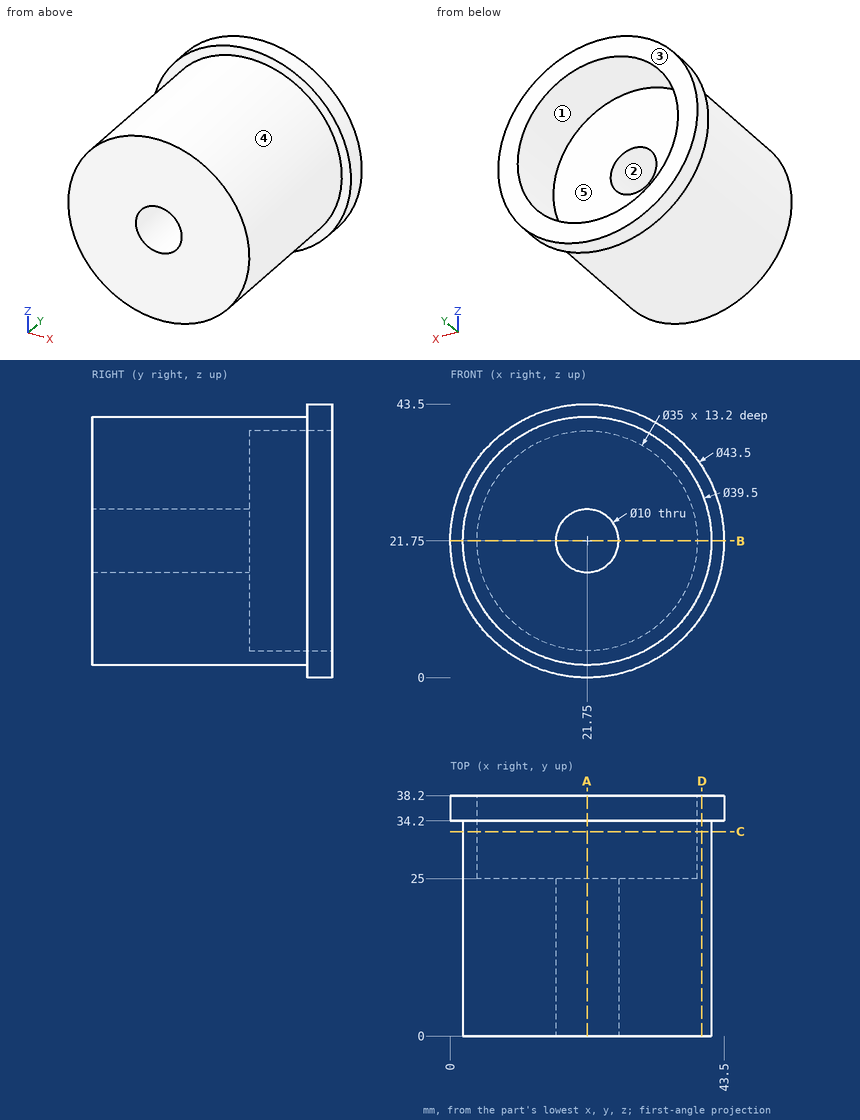
Geometry check sheet. Reference: drawing and pictorial views, mm from the part's lowest x, y, z. A direction names the side the tool comes from. Give positions to 0.01 mm unless a question says otherwise; leave off trailing zeros. Loops run counter-clockwise (first coordinate to the right, second up) from the corner with the lowest first, then second, coordinate; pieces in that order, holes last. Notation, with made-up numbers: (43.25, -25.5) - (101.25, -25.5) arc R17 ccw to (101.25, -16.5) - close; hole circle Ø9 at (85.5, -20). An arc over 180 degrees is marked (long way). Use CSV: the item, a comma, the result in double quotes. Start each with the question number.
Q1. Section check D-D, the plane x = 40. Record the cut outline in (y, z).
Q2. Section check B-B, the plane z = 21.75. Record the cut outline in (x, y).
Q3. Section check C-C, the plane y = 32.5. Record the cut outline in (x, z), and give its area (3 significant figures).
Q4. Section check A-A, the plane x = 21.75. Record the cut outline in (y, z).
Q5. Scan lines: probe 1 along X at (y, z) = (31, 21.75); probe 2 along Y at (x, z) = (31, 14); probe 3 along X at (y, z) = (3.5, 22). Record each from-to range of solid material in increasing order. Write a range as from..to.
Q6. Release check for a two-part mould opening along X. For the marked faces 3, 4 and 5 record: +X half, -X half, draft (parallel to the pull), parting line (faces both ways), or undercut.
Q7. Go/stop test with flat-tipped pins: pin 1 Ø6 at (x, y) = (33, 34) entering from -Z; pin 2 Ø1 at (x, y) = (24.5, 7) entering from +Z; pin 3 Ø5 at (y, z) = (15, 9.5) entering from +X. Record where each tip stops, or that it passes through.
Q8. Access from +Z, -Z, +X, -X, +Y, -Y to the whole of each face (thin tool, end or side, straight path). Record for the marked faces 1 and 2.
Findings below:
1,outline,"(0, 14.2) - (34.2, 14.2) - (34.2, 9.92) - (38.2, 9.92) - (38.2, 33.58) - (34.2, 33.58) - (34.2, 29.3) - (0, 29.3) - close"
2,outline,"(0, 34.2) - (2, 34.2) - (2, 0) - (16.75, 0) - (16.75, 25) - (4.25, 25) - (4.25, 38.2) - (0, 38.2) - close; (26.75, 0) - (41.5, 0) - (41.5, 34.2) - (43.5, 34.2) - (43.5, 38.2) - (39.25, 38.2) - (39.25, 25) - (26.75, 25) - close"
3,outline,"circle Ø39.5 at (21.75, 21.75); hole circle Ø35 at (21.75, 21.75)"
3,area,"263 mm^2"
4,outline,"(0, 2) - (34.2, 2) - (34.2, 0) - (38.2, 0) - (38.2, 4.25) - (25, 4.25) - (25, 16.75) - (0, 16.75) - close; (0, 26.75) - (25, 26.75) - (25, 39.25) - (38.2, 39.25) - (38.2, 43.5) - (34.2, 43.5) - (34.2, 41.5) - (0, 41.5) - close"
5,probe 1,"x = 2..4.25, 39.25..41.5"
5,probe 2,"y = 0..25"
5,probe 3,"x = 2..16.76, 26.74..41.5"
6,face 3,"draft"
6,face 4,"parting line"
6,face 5,"undercut"
7,pin 1,"stops at z = 1.63"
7,pin 2,"stops at z = 41.37"
7,pin 3,"stops at x = 38.93"
8,face 1,"+Y"
8,face 2,"+Y, -Y"
